Design review of the part shown in the three views and the two pictorial views. Dimensions are in mm from the part's minimum x, y and z. Coordinates: 2 decimals unless noted, no trailing zeros. Loops run counter-clockwise (first coordinate to the right, second up) from the corner with the lowest first, then second, coordinate; pieces in that order, holes last. Notation, with made-up numbers: (16, 52) - (68, 52) arc R15 ccw to (68, 80) - close; hole circle Ø5 at (79, 39.25). An arc over 180 degrees is marked (long way). One line per item, written item: value. Start each with the question number.
1. Insertion check: pin 1 (1.5 mm diameter, centred on x = 6.5, y = 0.5, fed in from -Z). The pin has a flat end and moves straight along its axis. Give the tip position at first contact, or say it passes through.
2. Take a section at A-A, the plane x = 3.5. State the section outline as (y, z) points, and give its area (3 significant figures).
3. To check wall thickness, follow line 1 (Y direction, x = 6.5, z = 1.8); line 2 (Y direction, x = 4, z = 2.45); line 3 (Z direction, x = 6.5, y = 0.2). State the ranges of each line that lie inside material, in increasing order. Write a range as from..to.
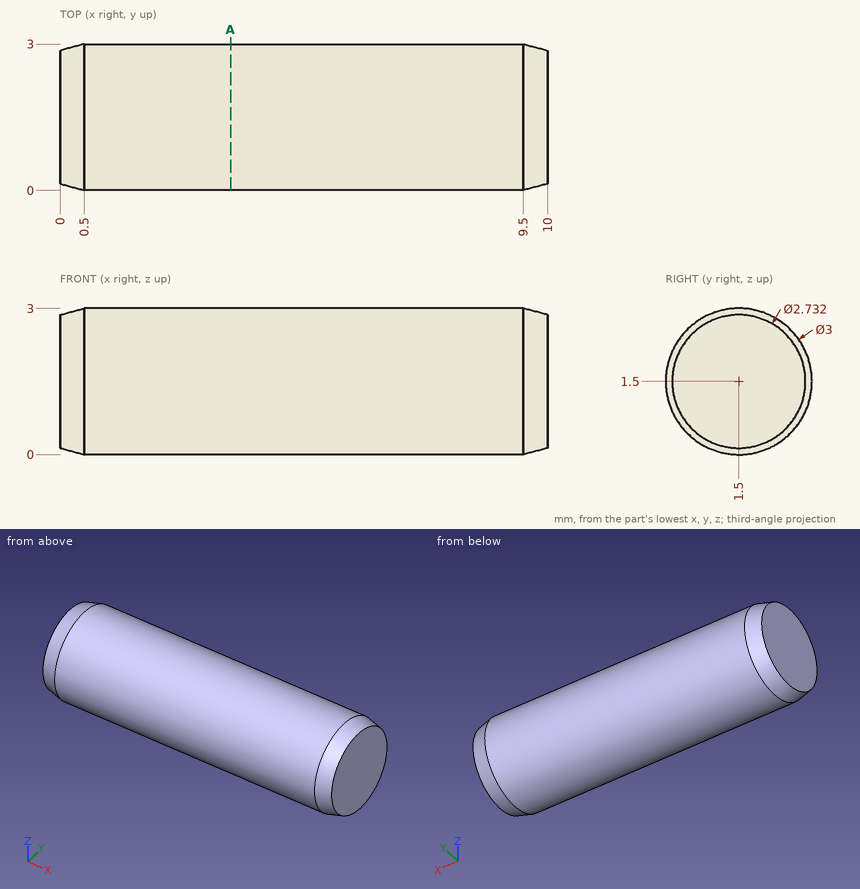
Solutions:
1. pin 1: z = 0.02
2. outline: circle Ø3 at (1.5, 1.5)
2. area: 7.07 mm2
3. line 1: 0.03..2.97
3. line 2: 0.34..2.66
3. line 3: 0.75..2.25
